```python
from build123d import *

# Parameters (mm, degrees)
BASE_FLANGE1_START      = -65
BASE_FLANGE1_DEPTH      = 130
CUT_EXTRUDE1_DEPTH      = 10
SKETCH4_R               = 4.25
CUT_EXTRUDE2_DEPTH      = 10
SKETCH5_R               = 3.175
SKETCH5_R_2             = 2.032
CUT_EXTRUDE3_DEPTH      = 10
CUT_EXTRUDE4_DEPTH      = 10
CHAMFER1_SIZE           = 10
EDGE_FLANGE1_DEPTH      = 140
EDGE_FLANGE1_BEND_DEPTH = 140
FILLET1_R               = 5
CHAMFER2_SIZE           = 10
SKETCH13_R              = 3
CUT_EXTRUDE5_DEPTH      = 10
SKETCH14_R              = 2.5
CUT_EXTRUDE6_DEPTH      = 236.837583095


# Read off the part's stored shape, not the designer's step: Base-Flange1
# Sheet-metal steps are written as plain solids
with BuildPart() as part:
    # Base-Flange1 outline → Base-Flange1 (new body)
    with BuildSketch(Plane.XY.offset(BASE_FLANGE1_START)):
        with BuildLine():
            Line((153.26, 5), (153.26, 15))
            Line((153.26, 15), (150, 15))
            Line((150, 15), (150, 5))
            ThreePointArc((150, 5), (148.535533906, 1.464466094), (145, 0))
            Line((145, 0), (5, 0))
            ThreePointArc((5, 0), (1.464466094, 1.464466094), (0, 5))
            Line((0, 5), (0, 95))
            ThreePointArc((0, 95), (1.464466094, 98.535533906), (5, 100))
            Line((5, 100), (30, 100))
            Line((30, 100), (30, 103.26))
            Line((30, 103.26), (5, 103.26))
            ThreePointArc((5, 103.26), (-0.840702013, 100.840702013), (-3.26, 95))
            Line((-3.26, 95), (-3.26, 5))
            ThreePointArc((-3.26, 5), (-0.840702013, -0.840702013), (5, -3.26))
            Line((5, -3.26), (145, -3.26))
            ThreePointArc((145, -3.26), (150.840702013, -0.840702013), (153.26, 5))
        make_face()
    extrude(amount=BASE_FLANGE1_DEPTH)

    # Sketch3 → Cut-Extrude1 (cut)
    with BuildSketch(Plane.ZY.offset(3.26)):
        with BuildLine():
            Line((-47, 35), (-47, 65))
            ThreePointArc((-47, 65), (-35, 77), (-23, 65))
            Line((-23, 65), (-23, 35))
            ThreePointArc((-23, 35), (-35, 23), (-47, 35))
        make_face()
        with BuildLine():
            Line((47, 35), (47, 65))
            ThreePointArc((47, 65), (35, 77), (23, 65))
            Line((23, 65), (23, 35))
            ThreePointArc((23, 35), (35, 23), (47, 35))
        make_face()
        with BuildLine():
            Line((12, 65), (12, 35))
            ThreePointArc((12, 35), (0, 23), (-12, 35))
            Line((-12, 35), (-12, 65))
            ThreePointArc((-12, 65), (0, 77), (12, 65))
        make_face()
    extrude(amount=-CUT_EXTRUDE1_DEPTH, mode=Mode.SUBTRACT)

    # Sketch4 → Cut-Extrude2 (cut)
    with BuildSketch(Plane(origin=(0, 103.26, 0), x_dir=(1, 0, 0), z_dir=(0, 1, 0))):
        with Locations(Location((17.5, 50, 0), (0, 0, 270))):
            Circle(SKETCH4_R)
        with Locations(Location((17.5, -50, 0), (0, 0, 270))):
            Circle(SKETCH4_R)
    extrude(amount=-CUT_EXTRUDE2_DEPTH, mode=Mode.SUBTRACT)

    # Sketch5 → Cut-Extrude3 (cut)
    with BuildSketch(Plane(origin=(0, 0, 0), x_dir=(1, 0, 0), z_dir=(0, 1, 0))):
        with Locations(Location((75, 0, 0), (0, 0, 270))):
            Circle(SKETCH5_R)
        with Locations(Location((75, 44.45, 0), (0, 0, 270))):
            Circle(SKETCH5_R_2)
        with Locations(Location((75, -44.45, 0), (0, 0, 270))):
            Circle(SKETCH5_R_2)
    extrude(amount=-CUT_EXTRUDE3_DEPTH, mode=Mode.SUBTRACT)

    # Sketch6 → Cut-Extrude4 (cut)
    with BuildSketch(Plane(origin=(0, 0, 0), x_dir=(1, 0, 0), z_dir=(0, 1, 0))):
        with BuildLine():
            Line((39.387502194, 8), (56.66969722, 8))
            ThreePointArc((56.66969722, 8), (75, 20), (93.33030278, 8))
            Line((93.33030278, 8), (110.612497806, 8))
            ThreePointArc((110.612497806, 8), (75, 36.5), (39.387502194, 8))
        make_face()
        with BuildLine():
            Line((110.612497806, -8), (93.33030278, -8))
            ThreePointArc((93.33030278, -8), (75, -20), (56.66969722, -8))
            Line((56.66969722, -8), (39.387502194, -8))
            ThreePointArc((39.387502194, -8), (75, -36.5), (110.612497806, -8))
        make_face()
    extrude(amount=-CUT_EXTRUDE4_DEPTH, mode=Mode.SUBTRACT)

    # Chamfer1
    chamfer1_edges = [part.edges().sort_by_distance(p)[0] for p in [
        (151.63, 15, -65),
        (151.63, 15, 65),
        (30, 101.63, -65),
        (30, 101.63, 65),
    ]]
    chamfer(chamfer1_edges, length=CHAMFER1_SIZE)

    # Edge-Flange1 section (across the edge) → Edge-Flange1 (add)
    with BuildSketch(Plane(origin=(5, 0, 70), x_dir=(0, 0, -1), z_dir=(1, 0, 0))):
        with BuildLine():
            Line((-3.26, 5), (-3.26, 15))
            Line((-3.26, 15), (0, 15))
            Line((0, 15), (0, 5))
            ThreePointArc((0, 5), (1.464466094, 1.464466094), (5, 0))
            Line((5, 0), (5, -3.26))
            ThreePointArc((5, -3.26), (-0.840702013, -0.840702013), (-3.26, 5))
        make_face()
    extrude(amount=EDGE_FLANGE1_DEPTH)

    # Edge-Flange1 section 2 (across the edge) → Edge-Flange1 bend (add)
    with BuildSketch(Plane(origin=(145, 0, -70), x_dir=(0, 0, 1), z_dir=(-1, 0, 0))):
        with BuildLine():
            Line((-3.26, 5), (-3.26, 15))
            Line((-3.26, 15), (0, 15))
            Line((0, 15), (0, 5))
            ThreePointArc((0, 5), (1.464466094, 1.464466094), (5, 0))
            Line((5, 0), (5, -3.26))
            ThreePointArc((5, -3.26), (-0.840702013, -0.840702013), (-3.26, 5))
        make_face()
    extrude(amount=EDGE_FLANGE1_BEND_DEPTH)

    # Fillet1
    fillet1_edges = [part.edges().sort_by_distance(p)[0] for p in [
        (56.66969722, -1.63, 8),
        (93.33030278, -1.63, 8),
        (110.612497806, -1.63, 8),
        (39.387502194, -1.63, 8),
        (93.33030278, -1.63, -8),
        (56.66969722, -1.63, -8),
        (39.387502194, -1.63, -8),
        (110.612497806, -1.63, -8),
    ]]
    fillet(fillet1_edges, radius=FILLET1_R)

    # Chamfer2
    chamfer2_edges = [part.edges().sort_by_distance(p)[0] for p in [
        (145, 15, -71.63),
        (145, 15, 71.63),
    ]]
    chamfer(chamfer2_edges, length=CHAMFER2_SIZE)

    # Sketch13 → Cut-Extrude5 (cut)
    with BuildSketch(Plane(origin=(0, 0, 0), x_dir=(0, 0, -1), z_dir=(1, 0, 0))):
        with Locations((-55, 47.196639222)):
            Circle(SKETCH13_R)
        with Locations((55, 47.196639222)):
            Circle(SKETCH13_R)
    extrude(amount=-CUT_EXTRUDE5_DEPTH, mode=Mode.SUBTRACT)

    # Sketch14 → Cut-Extrude6 (cut, through all)
    with BuildSketch(Plane.XY.offset(73.26)):
        with Locations((80, 10)):
            Circle(SKETCH14_R)
    extrude(amount=-CUT_EXTRUDE6_DEPTH, mode=Mode.SUBTRACT)


solid = part.part
```
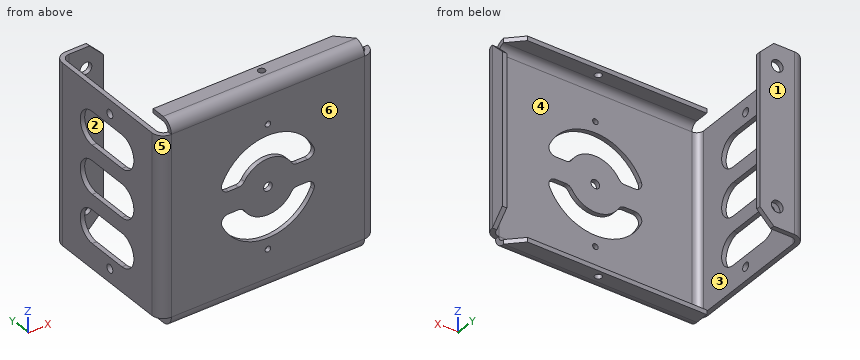
Geometry: final body of the model. Coordinates: model frame, mm. Face numbers are marked on the shaded views. A direction names the side the tool comes from. Round coordinates to 2 decimals unless told otherwise and drop trailing zeros. Write each loop counter-clockwise with the first axis right and the second up, starting at its lowest first coordinate (ties: lowest second). Pieces come first, ordered by that corner, then holes.
Item 1: Section query B-B (z = -50). Return loops of the section in (x, y).
Item 2: Mould query, pull axis X, two halves, no side actions, for the marked faces 4, 5 and 6. Classes: +X half, -X half, draft (parallel to the pull), parting line (faces both ways), or undercut.
Item 3: Section query A-A (x = 75). Give the number of separate pieces and of enclosed holes in the cut face, plus the area to 3 significant figures.
Item 4: Material intervals for L1, parallel to Z at x = 76.5, y = 6; L2, parallel to X at y = 13.5, z = -36; L3, parallel to Y at x = 128, z = -46, sorted ascending.
Item 5: Pin query (flat end, axial travel): P1, Ø1.6, axis at x = -1.5, y = 51, coming from the -Z side; P2, Ø7, axis at y = 47.2, z = 55, coming from the -X side; P3, Ø6.5, axis at x = 150, y = 1.5, coming from the +Z side; P4, Ø6.5, axis at y = 3.5, z = -70, coming from the -X side. Return the tip coordinate at first contact, or that it passes through.
Item 6: Section query D-D (x = 122.5). Return loops of the section in (y, z), plus the area to 3 significant figures.
Item 7: Section query C-C (y = 61.5). Return loops of the section in (x, z), plus the area to 3 significant figures.
Item 8: Set-up query: the marked faces 1, 2 and 3. Return all of +Z, -Z, +X, -X, +Y, -Y with unobstructed straight access to the full face (end or side cutting, diameter ignored); none if empty.
Completed:
1. outline: (-3.26, 5) arc R8.26 ccw to (5, -3.26) - (145, -3.26) arc R8.26 ccw to (153.26, 5) - (153.26, 15) - (150, 15) - (150, 5) arc R5 cw to (145, 0) - (5, 0) arc R5 cw to (0, 5) - (0, 95) arc R5 cw to (5, 100) - (13.25, 100) - (13.25, 103.26) - (5, 103.26) arc R8.26 ccw to (-3.26, 95) - close; (21.75, 100) - (30, 100) - (30, 103.26) - (21.75, 103.26) - close
2. face 4: undercut
2. face 5: -X half
2. face 6: draft
3. separate pieces: 6
3. enclosed holes: 0
3. area: 402 mm2
4. L1: z = -73.26 to -70, 70 to 73.26
4. L2: x = -3.26 to 0, 150 to 153.26
4. L3: y = -3.26 to 0
5. P1: stops at z = -65
5. P2: stops at x = -3.26
5. P3: stops at z = 65
5. P4: stops at x = 5
6. outline: (-3.26, -65) arc R8.26 ccw to (5, -73.26) - (15, -73.26) - (15, -70) - (5, -70) arc R5 cw to (0, -65) - (0, 65) arc R5 cw to (5, 70) - (15, 70) - (15, 73.26) - (5, 73.26) arc R8.26 ccw to (-3.26, 65) - close
6. area: 557 mm2
7. outline: (-3.26, -65) - (0, -65) - (0, -47) - (-3.26, -47) - close; (-3.26, -23) - (0, -23) - (0, -12) - (-3.26, -12) - close; (-3.26, 12) - (0, 12) - (0, 23) - (-3.26, 23) - close; (-3.26, 47) - (0, 47) - (0, 65) - (-3.26, 65) - close
7. area: 189 mm2
8. face 1: +Z, -Z, +X, -X, +Y
8. face 2: +Z, -Z, +X
8. face 3: +Z, -Z
